Autodesk Inventor part; units mm, degrees
ref_plane "YZ Plane" through (0, 0, 0) normal (1, 0, 0) x (0, 1, 0)
ref_plane "XZ Plane" through (0, 0, 0) normal (0, 1, 0) x (-1, 0, 0)
ref_plane "XY Plane" through (0, 0, 0) normal (0, 0, 1) x (1, 0, 0)
sketch "Sketch1" plane through (0, 0, 0) normal (0, 0, 1) x (1, 0, 0)
  line L0 (0, 0) -> (-6.5, 0)
  line L1 (-6.5, 0) -> (-6.5, -30)
  line L2 (-6.5, 0) -> (23.5, 0) construction
  line L3 (0, 0) -> (0, -30)
  line L4 (3, 0) -> (3, -30)
  line L5 (0, 3) -> (-9.5, 3)
  line L6 (-9.5, 3) -> (-9.5, -30)
  line L7 (3, -30) -> (0, -30)
  line L8 (-6.5, -30) -> (-9.5, -30)
  line L9 (28.4, 0) -> (71.8667, 11.6469)
  line L10 (28.4, 0) -> (73.4, 0) construction
  line L11 (28.4, 0) -> (3, 0)
  line L12 (0, 3) -> (28.005, 3)
  line L13 (71.0902, 14.5446) -> (28.005, 3)
  line L14 (71.8667, 11.6469) -> (71.0902, 14.5446)
  dimension "d0" = 6.5
  dimension "d1" = 30
  dimension "d2" = 90
  dimension "d3" = 30
  dimension "d4" = 3
  dimension "d5" = 3
  dimension "d6" = 25.4
  dimension "d7" = 45
  dimension "d8" = 15
extrude "Extrusion1" add sketch "Sketch1" along normal blind 68
sketch "Sketch2" plane through (71.8667, 11.6469, 0) normal (0.2588, -0.9659, 0) x (0.9659, 0.2588, 0)
  line L0 (0, 0) -> (-44.605, 0) construction
  line L1 (-22.3025, 0) -> (-22.3025, 68) construction
  line L2 (0, 68) -> (-44.605, 68) construction
  circle A0 centre (-22.3025, 34) radius 25.4 construction
  circle A1 centre (-22.3025, 8.6) radius 1.85
  circle A2 centre (-22.3025, 59.4) radius 1.85
  line L3 (-5.8525, 50.45) -> (-38.7525, 50.45)
  line L4 (-38.7525, 50.45) -> (-38.7525, 17.55)
  line L5 (-38.7525, 17.55) -> (-5.8525, 17.55)
  line L6 (-5.8525, 17.55) -> (-5.8525, 50.45)
  line L7 (-5.8525, 50.45) -> (-38.7525, 17.55) construction
  line L8 (-38.7525, 50.45) -> (-5.8525, 17.55) construction
  point P0 (-72.4323, 0)
  dimension "d12" = 50.8
  dimension "d13" = 3.7
  dimension "d14" = 3.7
  dimension "d15" = 32.9
  dimension "d16" = 32.9
extrude "Extrusion2" cut sketch "Sketch2" against normal blind 68
sketch "Sketch3" plane through (-9.5, -30, 0) normal (-1, 0, 0) x (0, 0, 1)
  line L0 (0, 33) -> (0, 0) construction
  line L1 (0, 16.5) -> (68, 16.5) construction
  line L2 (68, 33) -> (68, 0) construction
  circle A0 centre (34, 16.5) radius 1.85
  circle A1 centre (46.7, 16.5) radius 1.85
  circle A2 centre (21.3, 16.5) radius 1.85
  circle A3 centre (59.4, 16.5) radius 1.85
  circle A4 centre (8.6, 16.5) radius 1.85
  point P0 (0, 30)
  dimension "d19" = 3.7
  dimension "d22" = 12.7
extrude "Extrusion3" cut sketch "Sketch3" against normal blind 68
fillet "Fillet1" radius 8 2 edges at (71.4784, 13.0957, 0) (71.4784, 13.0957, 68)
fillet "Fillet2" radius 3 4 edges at (1.5, -30, 68) (-8, -30, 68) (1.5, -30, 0) (-8, -30, 0)
fillet "Fillet3" radius 0.6 25 edges at (-9.5, 3, 34) (-9.5, -29.1213, 67.1213) (-9.5, -30, 34) (-9.5, -29.1213, 0.8787) (-9.5, -12, 0) (-9.5, -12, 68) (9.2525, 3, 68) (9.2525, 3, 0) (68.8269, 13.9382, 2.3431) (71.0902, 14.5446, 34) (68.8269, 13.9382, 65.6569) (45.6839, 7.737, 68) (45.6839, 7.737, 0) (69.6034, 11.0404, 65.6569) (71.8667, 11.6469, 34) (69.6034, 11.0404, 2.3431) (46.2696, 4.7882, 0) (46.2696, 4.7882, 68) (15.7, 0, 68) (15.7, 0, 0) (3, -29.1213, 67.1213) (3, -13.5, 68) (3, -29.1213, 0.8787) (3, -13.5, 0) (3, -30, 34)
chamfer "Chamfer1" [suppressed]
properties part number "CamMountThrify"
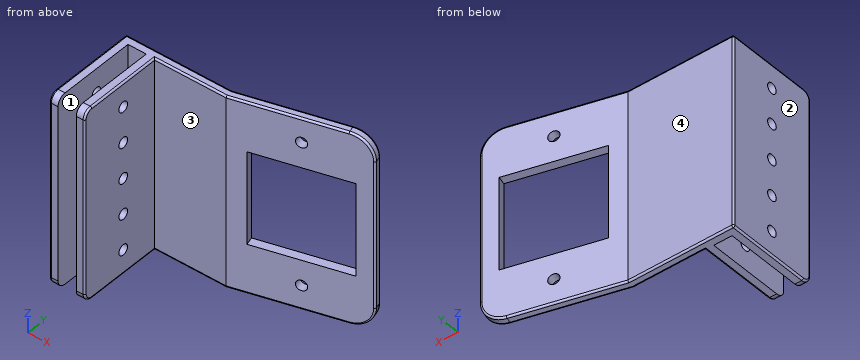
Part model, mm, in its own coordinate system. Face numbers are marked on the shaded views. A direction names the side the tool comes from. Coordinates: 2 decimals unless noted, no trailing zeros. Write each loop counter-clockwise with the first axis right and the second up, starting at its lowest first coordinate (ties: lowest second). Pieces come first, ordered by that corner, then holes. Notation, with made-up numbers: (-17, 67.25) - (6, 67.25) arc R36 cw to (6, 104.25) - close; hole circle Ø3 at (16.5, 42.25). An arc over 180 degrees is marked (long way). Put each result on its own line as item: value.
1. Band-saw the part on A-A (y = -26). Write the cut outline in (x, z).
Final values:
outline: (-9.5, 0.6) arc R0.6 ccw to (-8.9, 0) - (-6.5, 0) - (-6.5, 68) - (-8.9, 68) arc R0.6 ccw to (-9.5, 67.4) - close; (0, 0) - (2.4, 0) arc R0.6 ccw to (3, 0.6) - (3, 67.4) arc R0.6 ccw to (2.4, 68) - (0, 68) - close
2. Probe line 1 along Y through (x, z) = (1.25, 34); line 2 along X through (y, z) = (-23, 36.5); line 3 along Z through (x, y) = (-8, -13). List the from-to ranges inside material, lowest first. Write a range as [from, to].
Final values:
line 1: y = [-30, -15.35], [-11.65, 3]
line 2: x = [-9.5, -6.5], [0, 3]
line 3: z = [0, 6.82], [10.38, 19.52], [23.08, 32.22], [35.78, 44.92], [48.48, 57.62], [61.18, 68]
3. Band-saw the part on C-C (x = 17). Write the cut outline in (y, z).
Final values:
outline: (0, 0.6) arc R0.6 ccw to (0.6, 0) - (2.4, 0) arc R0.6 ccw to (3, 0.6) - (3, 67.4) arc R0.6 ccw to (2.4, 68) - (0.6, 68) arc R0.6 ccw to (0, 67.4) - close
4. Band-saw the part on B-B (z = 40). Write the cut outline in (x, y) (1 decimal), then the cut area to 3 significant figures.
Final values:
outline: (-9.5, -29.4) arc R0.6 ccw to (-8.9, -30) - (-6.5, -30) - (-6.5, 0) - (0, 0) - (0, -30) - (2.4, -30) arc R0.6 ccw to (3, -29.4) - (3, 0) - (28.4, 0) - (34.4, 1.6) - (33.7, 4.5) - (28, 3) - (-8.9, 3) arc R0.6 ccw to (-9.5, 2.4) - close; (65.4, 13) - (66.2, 10.1) - (71.3, 11.5) arc R0.6 ccw to (71.7, 12.2) - (71.2, 14) arc R0.6 ccw to (70.5, 14.4) - close
area: 328 mm²
5. Band-saw the part on D-D (z = 54). Write the cut outline in (x, y) (1 decimal), then the cut area to 3 significant figures.
Final values:
outline: (-9.5, -29.4) arc R0.6 ccw to (-8.9, -30) - (-6.5, -30) - (-6.5, 0) - (0, 0) - (0, -30) - (2.4, -30) arc R0.6 ccw to (3, -29.4) - (3, 0) - (28.4, 0) - (71.3, 11.5) arc R0.6 ccw to (71.7, 12.2) - (71.2, 14) arc R0.6 ccw to (70.5, 14.4) - (28, 3) - (-8.9, 3) arc R0.6 ccw to (-9.5, 2.4) - close
area: 427 mm²
6. 3-axis set-ups, long thin cutter, end or side, ignore diameter. For the marked faces 1, 2, 3 and 4: which of +Z, -Z, +X, -X, +Y, -Y reach the whole face in a straight line?
Final values:
face 1: +Z, -Z, -Y
face 2: +Z, -Z, -X, +Y, -Y
face 3: +Z, -Z, +X, -Y
face 4: +Z, -Z, -X, +Y
7. Flat gauge pins, fed straight in: pin 1 Ø8 at (y, z) = (-5, 7.5) entering from +X; pin 2 Ø4 at (x, z) = (24, 49.5) entering from +Y. Where does each tip first touch, or does it go through?
Final values:
pin 1: stops at x = 3
pin 2: stops at y = 3
